The listing builds one solid part. Answer for the finished solid, in the listing's coordinates (mm). A direction names the side the tool comes from. Give positions to 0.01 mm unless a question says otherwise; leave off trailing zeros. Write each loop counter-clockwise with the first axis right and the second up, starting at its lowest first coordinate (ties: lowest second). Pieces come first, ordered by that corner, then holes. Notation, with made-up numbers: (64, 18) - (103, 18) arc R23 cw to (103, 29) - close; hole circle Ø3 at (-9, 79). An arc over 180 degrees is marked (long way). One line per question, with ' | ' between items. Start each with the question number.
1. Given P1, Ø8, axis at x = 0, z = -20.5, coming from the -Y side; P2, Ø6, axis at y = 0, z = -29.5, coming from the -X side; P3, Ø8, axis at x = -4, y = 28.5, coming from the -Z side; P4, Ø1.5, axis at y = 7.5, z = -23, coming from the +X side, each flat-ended and moving along its own axis, determine where each tip first touches the part or whether it passes through.
2. For faces 5 (the face through (-9, 3, -20.523)), 6 (the face through (56, 1.524, -12)), 7 (the face through (53.035, -10.416, -28.567)), determine the directions among +Z, -Z, +X, -X, +Y, -Y from which every point of the face is accessible in a straight line to the end or side of a thin tool.
3. A cutting plane is placed at D-D (y = 6). Determine the outline of the cut face in (x, z), then the cut area to 3 significant figures.
4. A cutting plane is placed at C-C (z = -32). Determine the outline of the cut face in (x, y).
5. A cutting plane is placed at B-B (x = 14.5). Determine the outline of the cut face in (y, z), then the cut area to 3 significant figures.
6. Find the intervals of material crossed by L1, parallel to Y at x = 26.5, z = -31; L2, parallel to Z at x = 17, y = 25.5; L3, parallel to X at y = 27.5, z = -35, in increasing order. Write a range as from..to.
7. The mould has two halves that part along X. Classify faces 1 (the face through (48.244, 3.134, -12.584)), 2 (the face through (-5.064, 3.134, -12.584)), 3 (the face through (53, 3, -2.54)), 4 (the face through (41.656, 24, -19)): +X half, -X half, draft (parallel to the pull), parting line (faces both ways), or undercut.
```python
from build123d import *

# Parameters (mm, degrees)
SKETCH1_W                = 43.18
SKETCH1_H                = 38.1
BOSS_EXTRUDE1_DEPTH      = 14.986
SKETCH3_W                = 40.132
SKETCH3_H                = 35.052
BOSS_EXTRUDE2_DEPTH      = 19.0754
SKETCH4_W                = 17.9832
SKETCH4_H                = 3.175
BOSS_EXTRUDE3_DEPTH      = 20.9042
SKETCH6_R                = 3.5052
CUT_EXTRUDE2_DEPTH       = 5.699
CHAMFER1_SIZE            = 1.79578
CHAMFER2_SIZE            = 1.79578
BOSS_EXTRUDE4_DEPTH      = 19.9898
BOSS_EXTRUDE4_DEPTH_BACK = 7.47522
BOSS_EXTRUDE5_DEPTH      = 19.9898


with BuildPart() as part:
    # Sketch1 → Boss-Extrude1 (new body)
    with BuildSketch(Plane(origin=(0, 0, 0), x_dir=(1, 0, 0), z_dir=(0, 1, 0))):
        with Locations((21.59, 19.05)):
            Rectangle(SKETCH1_W, SKETCH1_H)
    extrude(amount=BOSS_EXTRUDE1_DEPTH)

    # Sketch3 → Boss-Extrude2 (add)
    with BuildSketch(Plane(origin=(0, 14.986, 0), x_dir=(1, 0, 0), z_dir=(0, 1, 0))):
        with Locations((21.59, 19.05)):
            Rectangle(SKETCH3_W, SKETCH3_H)
    extrude(amount=BOSS_EXTRUDE2_DEPTH)

    # Sketch4 → Boss-Extrude3 (add)
    with BuildSketch(Plane.ZY):
        with Locations((-11.5316, 3.1115)):
            Rectangle(SKETCH4_W, SKETCH4_H)
    boss_extrude3 = extrude(amount=BOSS_EXTRUDE3_DEPTH)

    # Mirror1: Boss-Extrude3 across plane
    add(boss_extrude3.mirror(Plane(origin=(21.59, 0, 0), x_dir=(0, 0, 1), z_dir=(1, 0, 0))))

    # Sketch6 → Cut-Extrude2 (cut, through all)
    with BuildSketch(Plane(origin=(0, 4.699, 0), x_dir=(1, 0, 0), z_dir=(0, 1, 0))):
        with Locations((-8.4074, 11.5316)):
            Circle(SKETCH6_R)
    cut_extrude2 = extrude(amount=-CUT_EXTRUDE2_DEPTH, mode=Mode.SUBTRACT)

    # Mirror3: Cut-Extrude2 across plane
    add(cut_extrude2.mirror(Plane(origin=(21.59, 0, 0), x_dir=(0, 0, 1), z_dir=(1, 0, 0))), mode=Mode.SUBTRACT)

    # Chamfer1
    chamfer1_edges = [part.edges().sort_by_distance(p)[0] for p in [
        (64.0842, 3.1115, -20.5232),
        (64.0842, 3.1115, -2.54),
    ]]
    chamfer(chamfer1_edges, length=CHAMFER1_SIZE)

    # Chamfer2
    chamfer2_edges = [part.edges().sort_by_distance(p)[0] for p in [
        (-20.9042, 3.1115, -20.5232),
        (-20.9042, 3.1115, -2.54),
    ]]
    chamfer(chamfer2_edges, length=CHAMFER2_SIZE)

    # Sketch7 → Boss-Extrude4 (add, two sides)
    with BuildSketch(Plane(origin=(43.18, 0, 0), x_dir=(0, 0, -1), z_dir=(1, 0, 0))) as boss_extrude4_sk:
        with BuildLine():
            Line((34.0614, 9.144), (34.036, 9.144))
            ThreePointArc((34.036, 9.144), (29.491990403, 7.261809597), (27.6098, 2.7178))
            Line((27.6098, 2.7178), (27.6098, 0))
            Line((27.6098, 0), (38.1, 0))
            Line((38.1, 0), (38.1, 7.716375445))
            ThreePointArc((38.1, 7.716375445), (36.203151726, 8.776590802), (34.0614, 9.144))
        make_face()
        with BuildLine():
            ThreePointArc((40.4876, 2.7178), (39.860059231, 5.487564893), (38.1, 7.716375445))
            Line((38.1, 7.716375445), (38.1, 0))
            Line((38.1, 0), (27.6098, 0))
            Line((27.6098, 0), (27.6098, -3.7719))
            ThreePointArc((27.6098, -3.7719), (28.261339144, -6.594290394), (30.084100746, -8.845496946))
            Line((30.084100746, -8.845496946), (34.0487, -4.740034236))
            Line((34.0487, -4.740034236), (38.016880079, -8.849204998))
            ThreePointArc((38.016880079, -8.849204998), (39.836984495, -6.602164583), (40.4876, -3.7846))
            Line((40.4876, -3.7846), (40.4876, 2.7178))
        make_face()
        with BuildLine():
            Line((34.0487, -6.0198), (30.832652906, -9.350114257))
            ThreePointArc((30.832652906, -9.350114257), (32.384087518, -9.991907918), (34.0487, -10.2108))
            Line((34.0487, -10.2108), (34.0487, -6.0198))
        make_face()
        with BuildLine():
            ThreePointArc((34.0614, -10.2108), (35.721039602, -9.992791591), (37.268072877, -9.353558206))
            Line((37.268072877, -9.353558206), (34.0487, -6.0198))
            Line((34.0487, -6.0198), (34.0487, -10.2108))
            Line((34.0487, -10.2108), (34.0614, -10.2108))
        make_face()
        with BuildLine():
            Line((34.0487, -4.740034236), (30.084100746, -8.845496946))
            ThreePointArc((30.084100746, -8.845496946), (30.449522295, -9.110940462), (30.832652906, -9.350114257))
            Line((30.832652906, -9.350114257), (34.0487, -6.0198))
            Line((34.0487, -6.0198), (37.268072877, -9.353558206))
            ThreePointArc((37.268072877, -9.353558206), (37.651344537, -9.114547904), (38.016880079, -8.849204998))
            Line((38.016880079, -8.849204998), (34.0487, -4.740034236))
        make_face()
    extrude(amount=BOSS_EXTRUDE4_DEPTH)
    extrude(boss_extrude4_sk.sketch, amount=-BOSS_EXTRUDE4_DEPTH_BACK)

    # Sketch7_3 → Boss-Extrude5 (add)
    with BuildSketch(Plane(origin=(43.18, 0, 0), x_dir=(0, 0, -1), z_dir=(1, 0, 0))):
        Polygon((34.0487, -4.740034236), (27.007269754, -12.031648709), (27.646762836, -12.6492), (34.0487, -6.0198), (40.450637164, -12.6492), (41.090130246, -12.031648709), align=None)
    extrude(amount=BOSS_EXTRUDE5_DEPTH)


solid = part.part
```
Determined:
1) P1: y = 0 | P2: x = 0 | P3: through | P4: x = 43.18
2) face 5: -Z, -X, +Y, -Y | face 6: +Z, +X, -Y | face 7: +Z, +X, -X
3) outline: (0, -38.1) - (35.7, -38.1) - (35.7, -39.59) - (63.17, -39.59) - (63.17, -28.51) - (43.18, -28.51) - (43.18, 0) - (0, 0) - close | area: 1,880 mm2
4) outline: (0, 0) - (35.7, 0) - (35.7, -9.88) - (63.17, -9.88) - (63.17, 8.81) - (43.18, 8.81) - (43.18, 14.99) - (41.66, 14.99) - (41.66, 34.06) - (1.52, 34.06) - (1.52, 14.99) - (0, 14.99) - close
5) outline: (0, -38.1) - (14.99, -38.1) - (14.99, -36.58) - (34.06, -36.58) - (34.06, -1.52) - (14.99, -1.52) - (14.99, 0) - (0, 0) - close | area: 1,240 mm2
6) L1: 0..34.06 | L2: -36.58..-1.52 | L3: 1.52..41.66
7) face 1: undercut | face 2: undercut | face 3: draft | face 4: +X half
